```python
from build123d import *

# Parameters (mm, degrees)
F1_DEPTH      = 30
F3_START      = 15.5
F2_R          = 12.75
F3_DEPTH      = 30
F4_R          = 7.5
F5_DEPTH      = 25
F5_DEPTH_BACK = 25
F6_R          = 11.75
F7_DEPTH      = 28
F8_R          = 1.55
F9_DEPTH      = 10
F14_R         = 2.1
F15_DEPTH     = 2
F16_R         = 1.5
F17_DEPTH     = 2.4
F18_R         = 1


# Not quite as in the source:
# - a fillet or chamfer that OpenCascade refuses, or shapes differently, is made with other operations: its cross-section is extruded or revolved along the edge and cut away or added


with BuildPart() as f1:
    # F0 (on Top) → F1 (new body)
    with BuildSketch(Plane.XY):
        with BuildLine():
            Line((7.7707002638, -18.4286792096), (7.7707002638, 18.4286792096))
            ThreePointArc((7.7707002638, 18.4286792096), (3.963988888, 19.6032342254), (0, 20))
            ThreePointArc((0, 20), (-20, 0), (0, -20))
            ThreePointArc((0, -20), (3.963988888, -19.6032342254), (7.7707002638, -18.4286792096))
        make_face()
        with BuildLine():
            Line((7.7707002638, 18.4286792096), (7.7707002638, 20))
            Line((7.7707002638, 20), (0, 20))
            ThreePointArc((0, 20), (3.963988888, 19.6032342254), (7.7707002638, 18.4286792096))
        make_face()
        with BuildLine():
            Line((0, -20), (7.7707002638, -20))
            Line((7.7707002638, -20), (7.7707002638, -18.4286792096))
            ThreePointArc((7.7707002638, -18.4286792096), (3.963988888, -19.6032342254), (0, -20))
        make_face()
        with BuildLine():
            Line((15.7707002638, 12), (16, 12))
            ThreePointArc((16, 12), (12.3123323076, 15.7609159996), (7.7707002638, 18.4286792096))
            Line((7.7707002638, 18.4286792096), (7.7707002638, -18.4286792096))
            ThreePointArc((7.7707002638, -18.4286792096), (12.3123323076, -15.7609159996), (16, -12))
            Line((16, -12), (15.7707002638, -12))
            Line((15.7707002638, -12), (15.7707002638, 12))
        make_face()
        with BuildLine():
            ThreePointArc((28.1113855937, -20), (30.4920884675, -16.1394715183), (32.3457879793, -12))
            Line((32.3457879793, -12), (16, -12))
            ThreePointArc((16, -12), (12.3123323076, -15.7609159996), (7.7707002638, -18.4286792096))
            Line((7.7707002638, -18.4286792096), (7.7707002638, -20))
            Line((7.7707002638, -20), (28.1113855937, -20))
        make_face()
        with BuildLine():
            ThreePointArc((20, 0), (18.973665961, 6.3245553203), (16, 12))
            Line((16, 12), (15.7707002638, 12))
            Line((15.7707002638, 12), (15.7707002638, -12))
            Line((15.7707002638, -12), (16, -12))
            ThreePointArc((16, -12), (18.973665961, -6.3245553203), (20, 0))
        make_face()
        with BuildLine():
            Line((16, 12), (32.3457879793, 12))
            ThreePointArc((32.3457879793, 12), (30.4920884675, 16.1394715183), (28.1113855937, 20))
            Line((28.1113855937, 20), (7.7707002638, 20))
            Line((7.7707002638, 20), (7.7707002638, 18.4286792096))
            ThreePointArc((7.7707002638, 18.4286792096), (12.3123323076, 15.7609159996), (16, 12))
        make_face()
        with BuildLine():
            Line((32.3457879793, 12), (40.7707002638, 12))
            ThreePointArc((40.7707002638, 12), (39.3392377906, 16.0833569274), (37.5, 20))
            Line((37.5, 20), (28.1113855937, 20))
            ThreePointArc((28.1113855937, 20), (30.4920884675, 16.1394715183), (32.3457879793, 12))
        make_face()
        with BuildLine():
            Line((28.1113855937, 20), (37.5, 20))
            ThreePointArc((37.5, 20), (-42.5, 0), (37.5, -20))
            Line((37.5, -20), (28.1113855937, -20))
            ThreePointArc((28.1113855937, -20), (-34.5, 0), (28.1113855937, 20))
        make_face()
        with BuildLine():
            ThreePointArc((37.5, -20), (39.3392377906, -16.0833569274), (40.7707002638, -12))
            Line((40.7707002638, -12), (32.3457879793, -12))
            ThreePointArc((32.3457879793, -12), (30.4920884675, -16.1394715183), (28.1113855937, -20))
            Line((28.1113855937, -20), (37.5, -20))
        make_face()
        with BuildLine():
            Line((40.7707002638, -12), (40.7707002638, 12))
            Line((40.7707002638, 12), (32.3457879793, 12))
            ThreePointArc((32.3457879793, 12), (33.9571766, 6.0959131685), (34.5, 0))
            ThreePointArc((34.5, 0), (33.9571766, -6.0959131685), (32.3457879793, -12))
            Line((32.3457879793, -12), (40.7707002638, -12))
        make_face()
        with BuildLine():
            ThreePointArc((40.7707002638, -12), (42.0654535291, -6.0619814743), (42.5, 0))
            ThreePointArc((42.5, 0), (42.0654535291, 6.0619814743), (40.7707002638, 12))
            Line((40.7707002638, 12), (40.7707002638, -12))
        make_face()
    extrude(amount=F1_DEPTH)

    # F2 (on Right) → F3 (cut)
    with BuildSketch(Plane.YZ.offset(F3_START)):
        with Locations((0, 15)):
            Circle(F2_R)
    extrude(amount=F3_DEPTH, mode=Mode.SUBTRACT)

    # F4 (on Front) → F5 (cut, two sides)
    with BuildSketch(Plane.XZ) as f5_sk:
        with Locations((44.5, 15)):
            Circle(F4_R)
    extrude(amount=-F5_DEPTH, mode=Mode.SUBTRACT)
    extrude(f5_sk.sketch, amount=F5_DEPTH_BACK, mode=Mode.SUBTRACT)

    # F6 (on face) → F7 (cut)
    with BuildSketch(Plane.XY.offset(30)):
        Circle(F6_R)
    extrude(amount=-F7_DEPTH, mode=Mode.SUBTRACT)

    # F8 (on face) → F9 (cut)
    with BuildSketch(Plane.YZ.offset(15.5)):
        with Locations((0, 15)):
            Circle(F8_R)
    extrude(amount=-F9_DEPTH, mode=Mode.SUBTRACT)

    # F10 (on Front) → F11 (revolve)
    with BuildSketch(Plane.XZ):
        Polygon((0, 4.4), (0, 2), (4.65, 2), (2.1, 4.4), align=None)
    revolve(axis=Axis((0, 0, 6.6192487312), (0, 0, 1)))

    # F12 (on Front) → F13 (revolve, cut)
    with BuildSketch(Plane.XZ):
        with BuildLine():
            ThreePointArc((0, -9.9), (4.7022600949, -7.9522600949), (6.65, -3.25))
            ThreePointArc((6.65, -3.25), (4.7022600949, 1.4522600949), (0, 3.4))
            Line((0, 3.4), (0, -9.9))
        make_face()
    revolve(axis=Axis((0, 0, -3.25), (0, 0, -1)), mode=Mode.SUBTRACT)

    # F14 (on face) → F15 (join)
    with BuildSketch(Plane.XY.offset(4.4)):
        Circle(F14_R)
    extrude(amount=F15_DEPTH)

    # F16 (on face) → F17 (cut)
    with BuildSketch(Plane.XY.offset(6.4)):
        Circle(F16_R)
    extrude(amount=-F17_DEPTH, mode=Mode.SUBTRACT)

    # F18
    f18_edges = [f1.edges().sort_by_distance(p)[0] for p in [
        (-2.1, 0, 4.4),
        (-4.65, 0, 2),
    ]]
    fillet(f18_edges, radius=F18_R)

    # F19: chamfer of 0.4 on 1 edges, made by hand

    # F19_s1 → F19_t2 (revolve, cut)
    with BuildSketch(Plane.XZ):
        with BuildLine():
            Line((6.2028339317, -0.0077040086), (5.5986981628, 0.3241952337))
            Line((5.5986981628, 0.3241952337), (5.5919460169, 0.3199047179))
            ThreePointArc((5.5919460169, 0.3199047179), (5.6990064099, 0.1613765462), (5.7947443643, -0.0039097744))
            Line((5.7947443643, -0.0039097744), (5.8017238817, -0.008))
            ThreePointArc((5.8017238817, -0.008), (6.0022789067, -0.008), (6.2028339317, -0.0157040086))
            Line((6.2028339317, -0.0157040086), (6.2028339317, -0.0077040086))
        make_face()
    revolve(axis=Axis((0, 0, 0), (0, 0, 1)), mode=Mode.SUBTRACT)


solid = f1.part
```
The listing builds one solid part. Answer for the finished solid, in the listing's coordinates (mm). A direction names the side the tool comes from. Give positions to 0.01 mm unless a question says otherwise; leave off trailing zeros. Loops run counter-clockwise (first coordinate to the right, second up) from the corner with the lowest first, then second, coordinate; pieces in that order, holes last. Notation, with made-up numbers: (9.5, 12.25) - (43.5, 12.25) arc R25 ccw to (43.5, 47.25) - close; hole circle Ø8 at (86.25, 68). An arc over 180 degrees is marked (long way). Return JSON: item names as keys, results as strings. Group by question number.
1. Find section A-A (x = -8). Write down the section's boundary in (y, z), then the cut area to 3 significant figures.
2. Find section B-B (y = -16.5). Write down the section's boundary in (x, z), then the cut area to 3 significant figures.
3. Given pin 1 Ø4 at (x, z) = (-26.5, 26) entering from -Y; pin 2 Ø0.9 at (x, y) = (0.5, 0) entering from +Z; pin 3 Ø2.5 at (y, z) = (0, 15) entering from -X, each flat-ended and moving along its own axis, determine where each tip first touches the part or whether it passes through.
4. Straight lines are drawn through the part: line 1 (X direction, y = 0.5, z = 19); line 2 (X direction, y = -10, z = 23); line 3 (Y direction, x = 14, z = 15). For each, find the intervals that lie inside material, in ascending order. Write a range as [from, to].
5. Which of the six approach directions +Z, -Z, +X, -X, +Y, -Y give full straight-line access (tool end or side, diameter ignored) to faces 4 (the flat face through (15.5, 0, 12)), 5 (the flat face through (9, 1, 0)), 6 (the cylindrical face through (37, 16, 15)), 7 (the cylindrical face through (11.207, 3.529, 16.196)), 8 (the flat face through (24, -12, 5))?
6. Find section D-D (x = -32). Write down the section's boundary in (y, z), then the cut area to 3 significant figures.
7. Find section C-C (z = 15). Write down the section's boundary in (x, y).
8. Determine the mould class of faces 1 (the cylindrical face through (13.601, -0.202, 16.537)), 2 (the cylindrical face through (37, -16, 15)), 3 (the cylindrical face through (-1.5, 0.07, 5.22)) for opening direction X: pulls with the +X half, pulls with the -X half, needs draft (parallel to the pull), parting line crosses it, or undercut.
Verdict:
{
 "1": {"outline": "(-41.74, 0) - (-33.56, 0) - (-33.56, 30) - (-41.74, 30) - close; (-18.33, 0) - (18.33, 0) - (18.33, 30) - (8.61, 30) - (8.61, 2) - (-8.61, 2) - (-8.61, 30) - (-18.33, 30) - close; (33.56, 0) - (41.74, 0) - (41.74, 30) - (33.56, 30) - close", "area": "1,110 mm^2"},
 "2": {"outline": "(-39.17, 0) - (-30.3, 0) - (-30.3, 30) - (-39.17, 30) - close; (-11.3, 0) - (39.17, 0) - (39.17, 9.73) arc R7.5 cw to (39.17, 20.27) - (39.17, 30) - (-11.3, 30) - close", "area": "1,760 mm^2"},
 "3": {"pin 1": "stops at y = -34.73", "pin 2": "stops at z = 4", "pin 3": "stops at x = -42.5"},
 "4": {"line 1": "x = [-42.5, -34.5], [-19.99, -11.74], [11.74, 15.5]", "line 2": "x = [-41.31, -33.02], [-17.32, -6.17], [6.17, 17.32], [33.02, 41.31]", "line 3": "y = [-40.13, -31.53], [-20, -1.55], [1.55, 20], [31.53, 40.13]"},
 "5": {"face 4": "+X", "face 5": "-Z, +X, -X, +Y, -Y", "face 6": "+X, +Y, -Y", "face 7": "+Z", "face 8": "+Z, -Z"},
 "6": {"outline": "(-27.97, 0) - (-12.89, 0) - (-12.89, 30) - (-27.97, 30) - close; (12.89, 0) - (27.97, 0) - (27.97, 30) - (12.89, 30) - close", "area": "904 mm^2"},
 "7": {"outline": "(11.65, -1.55) arc R11.75 cw (long way) to (11.65, 1.55) - (15.5, 1.55) - (15.5, 12.75) - (37, 12.75) - (37, 20.91) arc R42.5 ccw (long way) to (37, -20.91) - (37, -12.75) - (15.5, -12.75) - (15.5, -1.55) - close; hole (0, -20) arc R20 cw to (0, 20) - (28.11, 20) arc R34.5 ccw (long way) to (28.11, -20) - close"},
 "8": {"face 1": "needs draft", "face 2": "pulls with the +X half", "face 3": "undercut"}
}
